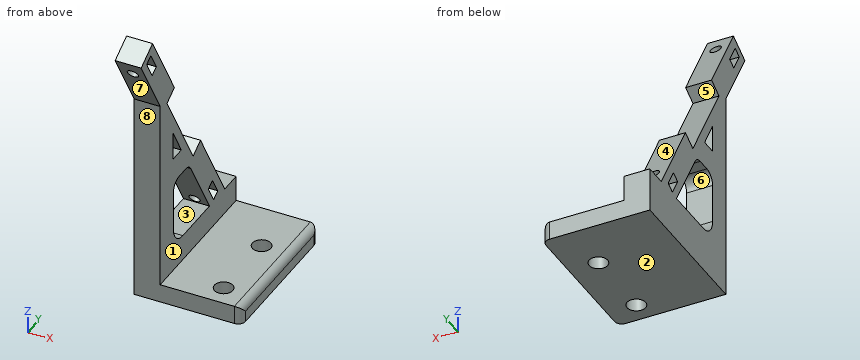
from build123d import *

# Parameters (mm, degrees)
BOSS_EXTRUDE1_DEPTH  = 7
SKETCH2_W            = 29
SKETCH2_H            = 40
SKETCH2_R            = 2.5
BOSS_EXTRUDE2_DEPTH  = 5
FILLET1_R            = 2
SKETCH3_R            = 1.5
CUT_EXTRUDE1_DEPTH   = 7.5
FILLET1_OF_MIRROR1_R = 2
SKETCH4_W            = 36.671322753
SKETCH4_H            = 72.42791828
CUT_EXTRUDE2_DEPTH   = 78.817930688


with BuildPart() as part:
    # Sketch1 → Boss-Extrude1 (new body)
    with BuildSketch(Plane(origin=(0, 0, 0), x_dir=(0, 0, -1), z_dir=(1, 0, 0))):
        Polygon((0, 0), (0, 40), (-7, 40), (-7, 34), (-29.083647797, 21.25), (-26.833647797, 17.352885683), (-50.649346401, 3.602885683), (-52.899346401, 7.5), (-72.817930688, -4), (-69.345498823, -10.014428415), (-52, 0), align=None)
        Polygon((-69.828328815, -4.926142338), (-64.848682743, -2.051142338), (-63.598682743, -4.216205848), (-68.578328815, -7.091205848), align=None, mode=Mode.SUBTRACT)
        Polygon((-39.949930688, 6.884), (-32.449930688, 11.134), (-32.449930688, 6.884), align=None, mode=Mode.SUBTRACT)
        with BuildLine():
            Line((-6.98, 25.947), (-6.98, 11.947))
            ThreePointArc((-6.98, 11.947), (-8.444466094, 8.411466094), (-11.98, 6.947))
            Line((-11.98, 6.947), (-22.48, 6.947))
            ThreePointArc((-22.48, 6.947), (-24.601320344, 7.825679656), (-25.48, 9.947))
            Line((-25.48, 9.947), (-25.48, 13.505607896))
            ThreePointArc((-25.48, 13.505607896), (-25.078135635, 15.007043949), (-23.98, 16.107))
            Line((-23.98, 16.107), (-6.98, 25.947))
        make_face(mode=Mode.SUBTRACT)
        Polygon((-13.512490144, 27.556681889), (-8.752389988, 30.311939862), (-7.5, 28.148257973), (-12.260100157, 25.393), align=None, mode=Mode.SUBTRACT)
    boss_extrude1 = extrude(amount=-BOSS_EXTRUDE1_DEPTH)

    # Sketch2 → Boss-Extrude2 (add)
    with BuildSketch(Plane(origin=(0, 0, 0), x_dir=(-1, 0, 0), z_dir=(0, 0, -1))):
        with Locations((14.5, 20)):
            Rectangle(SKETCH2_W, SKETCH2_H)
        with Locations((21.15335434, 25.78)):
            Circle(SKETCH2_R, mode=Mode.SUBTRACT)
        with Locations((21.15335434, 5.78)):
            Circle(SKETCH2_R, mode=Mode.SUBTRACT)
    boss_extrude2 = extrude(amount=BOSS_EXTRUDE2_DEPTH)

    # Fillet1
    fillet1_edges = [part.edges().sort_by_distance(p)[0] for p in [
        (-29, 20, 0),
        (-29, 0, -2.5),
        (-29, 40, -2.5),
    ]]
    fillet(fillet1_edges, radius=FILLET1_R)

    # Sketch3 → Cut-Extrude1 (cut)
    with BuildSketch(Plane(origin=(0, 28.531088913, 16.472431864), x_dir=(1, 0, 0), z_dir=(0, 0.866025404, 0.5))):
        with Locations((-3.5, 4.937822174)):
            Circle(SKETCH3_R)
        with Locations((-3.5, -60.062177826)):
            Circle(SKETCH3_R)
    cut_extrude1 = extrude(amount=-CUT_EXTRUDE1_DEPTH, mode=Mode.SUBTRACT)

    # Mirror1: Boss-Extrude1, Boss-Extrude2, Cut-Extrude1 across plane
    add(boss_extrude1.mirror(Plane(origin=(0, 0, 0), x_dir=(0, 0, 1), z_dir=(1, 0, 0))))
    add(boss_extrude2.mirror(Plane(origin=(0, 0, 0), x_dir=(0, 0, 1), z_dir=(1, 0, 0))))
    add(cut_extrude1.mirror(Plane(origin=(0, 0, 0), x_dir=(0, 0, 1), z_dir=(1, 0, 0))), mode=Mode.SUBTRACT)

    # Fillet1 of Mirror1
    fillet1_of_mirror1_edges = [part.edges().sort_by_distance(p)[0] for p in [
        (29, 20, 0),
        (29, 0, -2.5),
        (29, 40, -2.5),
    ]]
    fillet(fillet1_of_mirror1_edges, radius=FILLET1_OF_MIRROR1_R)

    # Sketch4 → Cut-Extrude2 (cut, through all)
    with BuildSketch(Plane(origin=(0, 0, -5), x_dir=(-1, 0, 0), z_dir=(0, 0, -1))):
        with Locations((18.335661377, 3.78604086)):
            Rectangle(SKETCH4_W, SKETCH4_H)
    extrude(amount=-CUT_EXTRUDE2_DEPTH, mode=Mode.SUBTRACT)


solid = part.part
Verification items for the finished model (mm, model axes). Face numbers are marked on the shaded views. A direction names the side the tool comes from. Coordinates: 2 decimals unless noted, no trailing zeros. Order: outer loops, then holes, each group sorted by start corner. A loop starts at its lowest first (then second) coordinate and runs counter-clockwise, first axis right, second up.
1. Sectioned sample at A-A, the plane y = 5.78. Record the cut outline in (x, z), and give its area (3 significant figures).
Results found:
outline: (0, -5) - (18.65, -5) - (18.65, 0) - (7, 0) - (7, 46.88) - (0, 46.88) - close; (0, 51.91) - (7, 51.91) - (7, 55.88) - (0, 55.88) - close; (23.65, -5) - (29, -5) - (29, -2) arc R2 ccw to (27, 0) - (23.65, 0) - close
area: 475 mm2
2. Sectioned sample at D-D, the plane y = 36. Record the cut outline in (x, z).
Results found:
outline: (0, -5) - (29, -5) - (29, -2) arc R2 ccw to (27, 0) - (7, 0) - (7, 7) - (0, 7) - close
3. Sectioned sample at C-C, the plane y = 14.5. Record the cut outline in (x, z) (3 decimals).
Results found:
outline: (0, -5) - (29, -5) - (29, -2) arc R2 ccw to (27, 0) - (7, 0) - (7, 6.98) - (0, 6.98) - close; (0, 25.311) - (7, 25.311) - (7, 31.775) - (0, 31.775) - close
4. Sectioned sample at B-B, the plane z = 20.5. Record the cut outline in (x, y).
Results found:
outline: (0, 0) - (7, 0) - (7, 6.95) - (0, 6.95) - close; (0, 18.12) - (7, 18.12) - (7, 26.21) - (0, 26.21) - close
5. Release check for a two-part mould opening along Z. For the marked faces 6, 7 and 8 record: +Z half, -Z half, draft (parallel to the pull), parting line (faces both ways), or undercut.
Results found:
face 6: undercut
face 7: -Z half
face 8: draft
6. Set-up check for the marked faces 1, 2, 3, 4 and 5: record each of +Z, -Z, +X, -X, +Y, -Y from which the full face is reachable in a straight line by a thin tool's end or side.
Results found:
face 1: +Z, +X, +Y, -Y
face 2: -Z, +X, -X, +Y, -Y
face 3: +X, -X
face 4: +Z, +X, -X, +Y
face 5: +X, -X, +Y
7. Scan lines: line 1 (Z direction, x = 14, y = 25); line 2 (X direction, y = 25, z = -3); line 3 (X direction, y = 17, z = 2). Record each from-to range of solid material in increasing order.
Results found:
line 1: z = -5 to 0
line 2: x = 0 to 18.78, 23.53 to 29
line 3: x = 0 to 7
8. Go/stop test with flat-tipped pins: pin 1 Ø5 at (x, y) = (18.5, 1) entering from +Z; pin 2 Ø4 at (x, z) = (5, 11.5) entering from +Y; pin 3 Ø1.3 at (x, y) = (2.5, 8) entering from +Z; pin 4 Ø6 at (x, y) = (21.15, 5.78) entering from -Z. Record where each tip stops, or that it passes through.
Results found:
pin 1: stops at z = 0
pin 2: stops at y = 32.56
pin 3: stops at z = 53.16
pin 4: stops at z = -5
